Could you check a few things on this drawing? It's one solid part, dimensions in mm from its lowest x, y, z. A direction names the side the tool comes from. Give positions to 0.01 mm unless a question says otherwise; leave off trailing zeros. Loops run counter-clockwise (first coordinate to the right, second up) from the corner with the lowest first, then second, coordinate; pieces in that order, holes last. Notation, with made-up numbers: (-33, 37) -> (-21, 37) arc R24 cw to (-21, 52) -> close; hole circle Ø8 at (10.5, -26). An arc over 180 degrees is marked (long way). One line per question, with ' | ' between items.
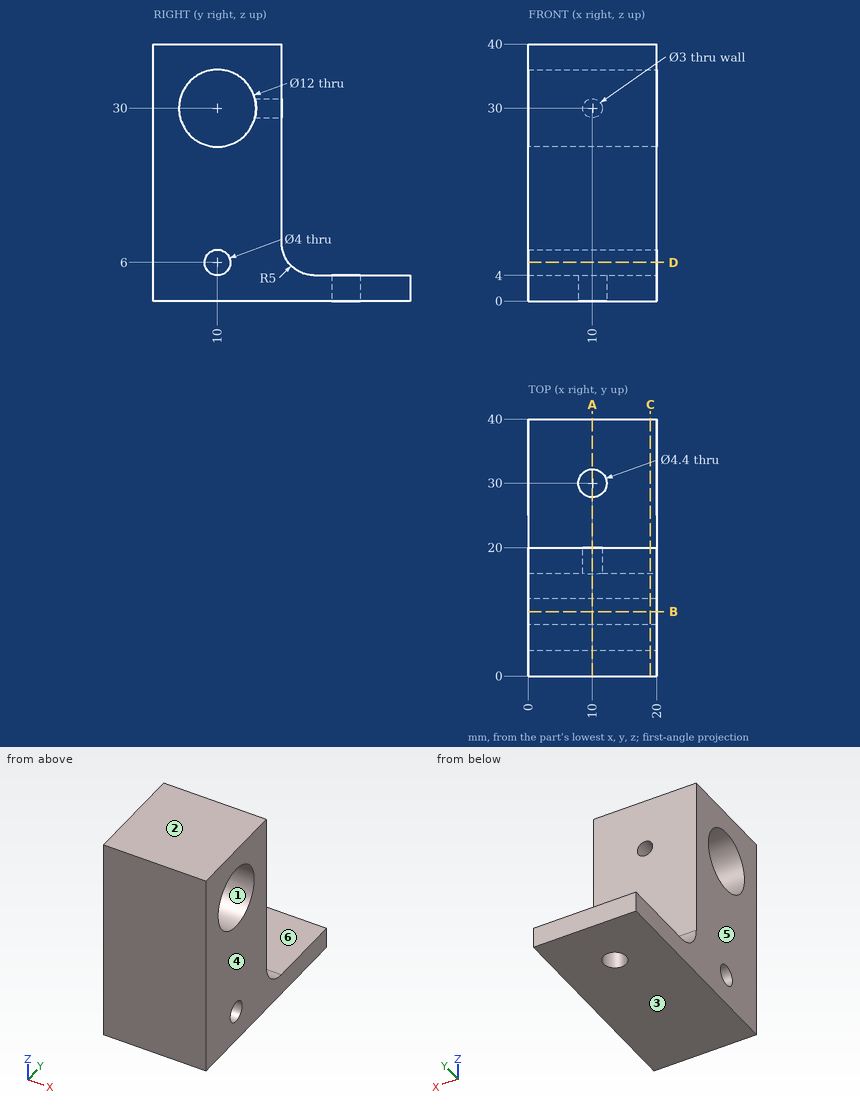
Q1. For pin 1 Ø2.5 at (x, y) = (10, 30) entering from +Z; pin 2 Ø2 at (x, y) = (14, 9.5) entering from -Z; pin 3 Ø5 at (x, z) = (2, 19) entering from +Y; pin 4 Ø10 at (x, y) = (11.5, 35) entering from +Z, each with a flat end and sliding along its axis, tell me the tip position at first contact or that it passes through.
Entries:
pin 1: through | pin 2: z = 0 | pin 3: y = 20 | pin 4: z = 4
Q2. If we section it at D-D (z = 6): Write out the boundary of the cut face in (x, y).
Entries:
outline: (0, 0) -> (20, 0) -> (20, 8) -> (0, 8) -> close; (0, 12) -> (20, 12) -> (20, 21) -> (0, 21) -> close
Q3. On a 3-axis mill with a long thin cutter (end or side, diameter ignored), from which of +Z, -Z, +X, -X, +Y, -Y can I reach the whole of each face in a straight line? I mean the marked faces 5 and 6. Say none if no direction works.
Entries:
face 5: +Z, -Z, -X, +Y, -Y | face 6: +Z, +X, -X, +Y
Q4. If I drill on probe 1 along X at (y, z) = (18.9, 30); probe 2 along Z at (x, y) = (10, 18.6); probe 3 along Y at (x, z) = (19, 20), over which ranges is the centre line in solid material (lowest first)? Write a range as from..to.
Entries:
probe 1: 0..8.5, 11.5..20 | probe 2: 0..28.5, 31.5..40 | probe 3: 0..20
Q5. If we section it at C-C (x = 19): Write out the boundary of the cut face in (y, z).
Entries:
outline: (0, 0) -> (40, 0) -> (40, 4) -> (25, 4) arc R5 cw to (20, 9) -> (20, 40) -> (0, 40) -> close; hole circle Ø12 at (10, 30); hole circle Ø4 at (10, 6)
Q6. If we section it at A-A (x = 10): Write out the boundary of the cut face in (y, z).
Entries:
outline: (0, 0) -> (27.8, 0) -> (27.8, 4) -> (25, 4) arc R5 cw to (20, 9) -> (20, 28.5) -> (15.81, 28.5) arc R6 cw (long way) to (15.81, 31.5) -> (20, 31.5) -> (20, 40) -> (0, 40) -> close; (32.2, 0) -> (40, 0) -> (40, 4) -> (32.2, 4) -> close; hole circle Ø4 at (10, 6)
Q7. If we mould it in two halves opening along Z, with no side actions, what happens to the marked faces 1, 2, 3 and 4? For each: pulls with the +Z half, pulls with the -Z half, needs draft (parallel to the pull), parting line crosses it, or undercut.
Entries:
face 1: undercut | face 2: pulls with the +Z half | face 3: pulls with the -Z half | face 4: needs draft
Q8. If we section it at B-B (y = 10): Write out the boundary of the cut face in (x, z), plus the area to 3 significant figures.
Entries:
outline: (0, 0) -> (20, 0) -> (20, 4) -> (0, 4) -> close; (0, 8) -> (20, 8) -> (20, 24) -> (0, 24) -> close; (0, 36) -> (20, 36) -> (20, 40) -> (0, 40) -> close | area: 480 mm²
